Read the model definition and answer for the solid it produces. Units are mm, in the model's axes. Give positions to 0.01 mm unless a question says otherwise; leave off trailing zeros. Loops run counter-clockwise (first coordinate to the right, second up) from the corner with the lowest first, then second, coordinate; pieces in that order, holes last. Notation, with made-up numbers: (50.5, 41) -> (66.5, 41) arc R27 cw to (66.5, 60) -> close; hole circle Ø11 at (-24.5, 31.5). An arc over 180 degrees is marked (long way). Write each question's results on one line, items separated by ' | '. Start each with the question number.
Item 1: Determine the mould class of faces 1 (the flat face through (-1, 8, 0)), 2 (the cylindrical face through (75, -133.57, 1.52)), 3 (the cylindrical face through (-75.07, -133.5, 1.52)), 4 (the cylindrical face through (-2.38, 120.5, 1.52)) for opening direction X: +X half, -X half, draft (parallel to the pull), parting line (faces both ways), or undercut.
Item 2: Section A-A on x = 0 is taken. Write down the section's boundary in (y, z), and give its area (3 significant figures).
Item 3: Section B-B on z = 2.4 is taken. State how many separate pieces and enclosed holes the cut face has, and give its area (3 significant figures).
Item 4: Section C-C on x = -44.5 is taken. Write down the section's boundary in (y, z) (3 decimals), and give its area (3 significant figures).
Item 5: This flat-tipped pin is pushed along its axis until it touches: P1, Ø4, axis at x = 19.05, y = 98.02, coming from the +Z side. Where does it stop, or does it pass through?
Item 6: Find the intervals of material crossed by line 1 (Y direction, x = 0, z = 2.15); line 2 (Y direction, x = -25, z = 1.85); line 3 (Y direction, x = 19.05, z = 1.45), in increasing order.
```python
from build123d import *

# Parameters (mm, degrees)
CROQUIS1_W              = 153
CROQUIS1_H              = 270
SALIENTE_EXTRUIR1_DEPTH = 3
CROQUIS2_R              = 2
CORTAR_EXTRUIR1_DEPTH   = 4
REDONDEO1_R             = 5
SALIENTE_EXTRUIR2_DEPTH = 3
REDONDEO2_R             = 25
REDONDEO3_R             = 10
CROQUIS5_R              = 11
CORTAR_EXTRUIR3_DEPTH   = 4
CROQUIS6_R              = 1.5
CROQUIS6_W              = 15
CROQUIS6_H              = 5
CORTAR_EXTRUIR4_DEPTH   = 4
CROQUIS7_R              = 1.5
CORTAR_EXTRUIR5_DEPTH   = 10


with BuildPart() as part:
    # Croquis1 → Saliente-Extruir1 (new body)
    with BuildSketch(Plane.XY):
        Rectangle(CROQUIS1_W, CROQUIS1_H)
    extrude(amount=SALIENTE_EXTRUIR1_DEPTH)

    # Croquis2 → Cortar-Extruir1 (cut, through all)
    with BuildSketch(Plane.XY.offset(3)):
        with Locations((-71.5, 41.5)):
            Circle(CROQUIS2_R)
        with Locations((-71.5, -61.5)):
            Circle(CROQUIS2_R)
        with Locations((71.5, -61.5)):
            Circle(CROQUIS2_R)
        with Locations((71.5, 41.5)):
            Circle(CROQUIS2_R)
    extrude(amount=-CORTAR_EXTRUIR1_DEPTH, mode=Mode.SUBTRACT)

    # Redondeo1
    redondeo1_edges = [part.edges().sort_by_distance(p)[0] for p in [
        (76.5, -135, 1.5),
        (-76.5, -135, 1.5),
        (-76.5, 135, 1.5),
        (76.5, 135, 1.5),
    ]]
    fillet(redondeo1_edges, radius=REDONDEO1_R)

    # Croquis4 → Saliente-Extruir2 (add)
    with BuildSketch(Plane.XY.offset(3)):
        Polygon((22, 147.2375), (-22, 147.2375), (-71.5, 135), (71.5, 135), align=None)
    extrude(amount=-SALIENTE_EXTRUIR2_DEPTH)

    # Redondeo2
    redondeo2_edges = [part.edges().sort_by_distance(p)[0] for p in [
        (-71.5, 135, 1.5),
        (71.5, 135, 1.5),
    ]]
    fillet(redondeo2_edges, radius=REDONDEO2_R)

    # Redondeo3
    redondeo3_edges = [part.edges().sort_by_distance(p)[0] for p in [
        (22, 147.2375, 1.5),
        (-22, 147.2375, 1.5),
    ]]
    fillet(redondeo3_edges, radius=REDONDEO3_R)

    # Croquis5 → Cortar-Extruir3 (cut, through all)
    with BuildSketch(Plane.XY.offset(3)):
        with Locations((0, 131.2375)):
            Circle(CROQUIS5_R)
    extrude(amount=-CORTAR_EXTRUIR3_DEPTH, mode=Mode.SUBTRACT)

    # Croquis6 → Cortar-Extruir4 (cut, through all)
    with BuildSketch(Plane.XY.offset(3)):
        with Locations((-8.89, 98.0200592)):
            Circle(CROQUIS6_R)
        with Locations((19.05, 98.0200592)):
            Circle(CROQUIS6_R)
        with Locations((24.13, 47.2200592)):
            Circle(CROQUIS6_R)
        with Locations((-24.13, 47.2200592)):
            Circle(CROQUIS6_R)
        with Locations((0, 23.297668012)):
            Rectangle(CROQUIS6_W, CROQUIS6_H)
    extrude(amount=-CORTAR_EXTRUIR4_DEPTH, mode=Mode.SUBTRACT)

    # Croquis7 → Cortar-Extruir5 (cut)
    with BuildSketch(Plane.XY.offset(3)):
        with Locations((-25, -89.038395192)):
            Circle(CROQUIS7_R)
        with Locations((25, -89.038395192)):
            Circle(CROQUIS7_R)
        with Locations((-25, -119.038395192)):
            Circle(CROQUIS7_R)
        with Locations((25, -119.038395192)):
            Circle(CROQUIS7_R)
    extrude(amount=-CORTAR_EXTRUIR5_DEPTH, mode=Mode.SUBTRACT)


solid = part.part
```
Findings:
1) face 1: draft | face 2: +X half | face 3: -X half | face 4: undercut
2) outline: (-135, 0) -> (20.8, 0) -> (20.8, 3) -> (-135, 3) -> close; (25.8, 0) -> (120.24, 0) -> (120.24, 3) -> (25.8, 3) -> close; (142.24, 0) -> (147.24, 0) -> (147.24, 3) -> (142.24, 3) -> close | area: 766 mm2
3) separate pieces: 1 | enclosed holes: 14 | area: 41,900 mm2
4) outline: (-135, 0) -> (141.675, 0) -> (141.675, 3) -> (-135, 3) -> close | area: 830 mm2
5) P1: z = 3
6) line 1: -135 to 20.8, 25.8 to 120.24, 142.24 to 147.24 | line 2: -135 to -120.54, -117.54 to -90.54, -87.54 to 46, 48.44 to 146.5 | line 3: -135 to 96.52, 99.52 to 147.24
